Autodesk Inventor part; units mm, degrees
ref_plane "YZ Plane" through (0, 0, 0) normal (1, 0, 0) x (0, 1, 0)
ref_plane "XZ Plane" through (0, 0, 0) normal (0, 1, 0) x (-1, 0, 0)
ref_plane "XY Plane" through (0, 0, 0) normal (0, 0, 1) x (1, 0, 0)
sketch "Sketch1" plane through (0, 0, 0) normal (0, 0, 1) x (1, 0, 0)
  line L0 (-7.5, -30) -> (7.5, -30)
  line L1 (7.5, -30) -> (7.5, 30)
  line L2 (7.5, 30) -> (-7.5, 30)
  line L3 (-7.5, 30) -> (-7.5, -30)
  line L4 (-7.5, -30) -> (7.5, 30) construction
  line L5 (7.5, -30) -> (-7.5, 30) construction
  line L6 (0, 30) -> (0, 22.5)
  circle A0 centre (0, 22.5) radius 5.25
  line L7 (0, -30) -> (0, -26)
  line L8 (-3, -26) -> (3, -26)
  circle A1 centre (-3, -26) radius 1.5
  circle A2 centre (3, -26) radius 1.5
  point P0 (0, 0)
  dimension "d0" = 15
  dimension "d1" = 60
  dimension "d2" = 7.5
  dimension "d3" = 10.5
  dimension "d6" = 4
  dimension "d7" = 6
  dimension "d8" = 3
  dimension "d9" = 3
extrude "Extrusion1" add sketch "Sketch1" against normal blind 1
chamfer "Chamfer1" distance 2 angle 45 4 edges at (7.5, 30, -0.5) (-7.5, 30, -0.5) (7.5, -30, -0.5) (-7.5, -30, -0.5)
properties part number "Loadcell_lever"
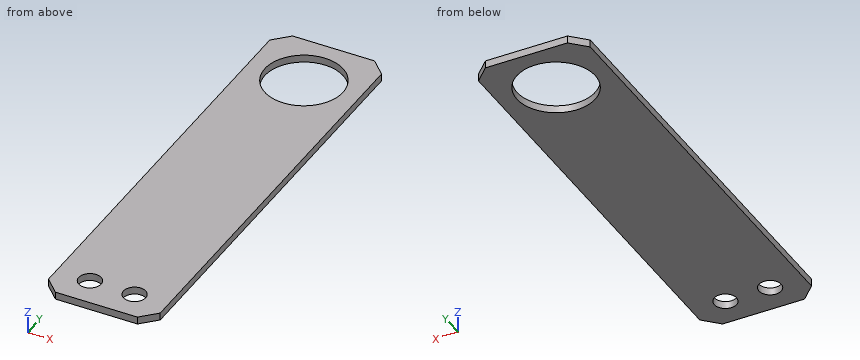
Part model, mm, in its own coordinate system. Round coordinates to 2 decimals unless told otherwise and drop trailing zeros. Loops run counter-clockwise (first coordinate to the right, second up) from the corner with the lowest first, then second, coordinate; pieces in that order, holes last. Notation, with made-up numbers: (-30.75, -32) -> (-10.75, -32) arc R17 cw to (-10.75, -20) -> close; hole circle Ø1 at (18.25, 62.5). An arc over 180 degrees is marked (long way). Use a Markdown table: item, result.
1) Cut at C-C, the plane z = -0.8. List the corners of the cut face in (x, y).
The answers:
| item | result |
|---|---|
| outline | (-7.5, -28) -> (-5.5, -30) -> (5.5, -30) -> (7.5, -28) -> (7.5, 28) -> (5.5, 30) -> (-5.5, 30) -> (-7.5, 28) -> close; hole circle Ø10.5 at (0, 22.5); hole circle Ø3 at (-3, -26); hole circle Ø3 at (3, -26) |
2) Probe line 1 (Y direction, x = -2, z = -0.05); line 2 (Y direction, x = -4, z = -0.3); line 3 (X direction, y = 22.5, z = -0.6). List the from-to ranges inside material, lowest first. Write a range as [from, to].
The answers:
| item | result |
|---|---|
| line 1 | y = [-30, -27.12], [-24.88, 17.65], [27.35, 30] |
| line 2 | y = [-30, -27.12], [-24.88, 19.1], [25.9, 30] |
| line 3 | x = [-7.5, -5.25], [5.25, 7.5] |
3) Cut at B-B, the plane x = 0. List the corners of the cut face in (y, z), and give its area (3 significant figures).
The answers:
| item | result |
|---|---|
| outline | (-30, -1) -> (17.25, -1) -> (17.25, 0) -> (-30, 0) -> close; (27.75, -1) -> (30, -1) -> (30, 0) -> (27.75, 0) -> close |
| area | 49.5 mm2 |
4) Cut at A-A, the plane y = -26. List the corners of the cut face in (x, z).
The answers:
| item | result |
|---|---|
| outline | (-7.5, -1) -> (-4.5, -1) -> (-4.5, 0) -> (-7.5, 0) -> close; (-1.5, -1) -> (1.5, -1) -> (1.5, 0) -> (-1.5, 0) -> close; (4.5, -1) -> (7.5, -1) -> (7.5, 0) -> (4.5, 0) -> close |
5) Cut at D-D, the plane y = 22.5. List the corners of the cut face in (x, z).
The answers:
| item | result |
|---|---|
| outline | (-7.5, -1) -> (-5.25, -1) -> (-5.25, 0) -> (-7.5, 0) -> close; (5.25, -1) -> (7.5, -1) -> (7.5, 0) -> (5.25, 0) -> close |
